Design review of the part built by this model. Coordinates are the model's own, in mm. A direction names the side the tool comes from. Coordinates: 2 decimals unless noted, no trailing zeros. Loops run counter-clockwise (first coordinate to the right, second up) from the corner with the lowest first, then second, coordinate; pieces in that order, holes last. Notation, with made-up numbers: (80, -18.75) -> (114, -18.75) arc R23 cw to (114, -2.75) -> close; hole circle Ø7 at (48, 8). An arc over 180 degrees is marked (long way). One line per item, written item: value. Start each with the question number.
1. Add section A-A on z = 11. Give the number of separate pieces and of enclosed holes in the cut face, plus the area to 3 significant figures.
2. Draft analysis for pull direction Y (two halves, no side actions). For faces 3 (the cylindrical face through (266.06, 1.81, 17.53)), 4 (the cylindrical face through (10.79, 10.89, 19.91)), 5 (the flat face through (136, 139.7, 18)), state which applies: pulls with the +Y half, pulls with the -Y half, needs draft (parallel to the pull), parting line crosses it, or undercut.
3. Add section B-B on y = 16. Write out the cut boundary in (x, z).
4. Insertion check: pin 1 (1.5 mm diameter, centred on x = 147.5, y = 18.5, fed in from +Z); pin 2 (1.5 mm diameter, centred on x = 6, z = 33.5, fed in from -Y); pin 3 (1.3 mm diameter, centred on y = 135, z = 25.5, fed in from -X); pin 4 (1.6 mm diameter, centred on x = 260.5, y = 6, fed in from +Z). Each pin has a flat end and moves straight along its axis. Give the tip position at first contact, or say it passes through.
5. For probe 1 along Y at (x, z) = (261.62, 12.5); probe 2 along Y at (x, z) = (198, 31); probe 3 along X at (y, z) = (133.35, 15.75), list the stretches that pass through material, from the lowest coordinate up.
6. Machinability: for faces 1 (the flat face through (136, 135.89, 19)), 2 (the cylindrical face through (1.91, 137.89, 17.53)), which of the approach directions +Z, -Z, +X, -X, +Y, -Y give a long, thin tool a straight path to every point of the face, cutting with its end or side? Answer none if there is none.
7. Add section C-C on x = 210. Write out the cut boundary in (y, z).
```python
from build123d import *

# Parameters (mm, degrees)
BOSS_EXTRUDE1_DEPTH = 35.56
SHELL1_T            = -3.81
BOSS_EXTRUDE2_REACH = 306.284
SKETCH2_R           = 1.5875
CUT_EXTRUDE1_DEPTH  = 5.08


with BuildPart() as part:
    # Sketch1 → Boss-Extrude1 (new body)
    with BuildSketch(Plane.XY):
        with BuildLine():
            Line((6.35, 0), (261.62, 0))
            ThreePointArc((261.62, 0), (266.110128061, 1.859871939), (267.97, 6.35))
            Line((267.97, 6.35), (267.97, 133.35))
            ThreePointArc((267.97, 133.35), (266.110128061, 137.840128061), (261.62, 139.7))
            Line((261.62, 139.7), (6.35, 139.7))
            ThreePointArc((6.35, 139.7), (1.859871939, 137.840128061), (0, 133.35))
            Line((0, 133.35), (0, 6.35))
            ThreePointArc((0, 6.35), (1.859871939, 1.859871939), (6.35, 0))
        make_face()
    extrude(amount=BOSS_EXTRUDE1_DEPTH)

    # Shell1
    shell1_openings = [part.faces().sort_by_distance(p)[0] for p in [
        (133.985, 69.85, 35.56),
    ]]
    offset(amount=SHELL1_T, openings=shell1_openings, kind=Kind.INTERSECTION)

    # Sketch2 → Boss-Extrude2 (add, up to next)
    with BuildSketch(Plane.XY.offset(35.56), mode=Mode.PRIVATE) as boss_extrude2_sk1:
        with BuildLine():
            Line((255.27, 139.7), (261.62, 139.7))
            ThreePointArc((261.62, 139.7), (266.110128061, 137.840128061), (267.97, 133.35))
            Line((267.97, 133.35), (267.97, 127))
            Line((267.97, 127), (261.62, 127))
            ThreePointArc((261.62, 127), (257.129871939, 128.859871939), (255.27, 133.35))
            Line((255.27, 133.35), (255.27, 139.7))
        make_face()
        with Locations(Location((261.62, 133.35, 0), (0, 0, 180))):
            Circle(SKETCH2_R, mode=Mode.SUBTRACT)
    boss_extrude2_tool1 = extrude(boss_extrude2_sk1.sketch, amount=-BOSS_EXTRUDE2_REACH, mode=Mode.PRIVATE) - part.part
    # Sketch2 → Boss-Extrude2 (add, up to next)
    with BuildSketch(Plane.XY.offset(35.56), mode=Mode.PRIVATE) as boss_extrude2_sk2:
        with BuildLine():
            Line((12.7, 133.35), (12.7, 139.7))
            Line((12.7, 139.7), (6.35, 139.7))
            ThreePointArc((6.35, 139.7), (1.859871939, 137.840128061), (0, 133.35))
            Line((0, 133.35), (0, 127))
            Line((0, 127), (6.35, 127))
            ThreePointArc((6.35, 127), (10.840128061, 128.859871939), (12.7, 133.35))
        make_face()
        with Locations((6.35, 133.35)):
            Circle(SKETCH2_R, mode=Mode.SUBTRACT)
    boss_extrude2_tool2 = extrude(boss_extrude2_sk2.sketch, amount=-BOSS_EXTRUDE2_REACH, mode=Mode.PRIVATE) - part.part
    # Sketch2 → Boss-Extrude2 (add, up to next)
    with BuildSketch(Plane.XY.offset(35.56), mode=Mode.PRIVATE) as boss_extrude2_sk3:
        with BuildLine():
            Line((12.7, 0), (6.35, 0))
            ThreePointArc((6.35, 0), (1.859871939, 1.859871939), (0, 6.35))
            Line((0, 6.35), (0, 12.7))
            Line((0, 12.7), (6.35, 12.7))
            ThreePointArc((6.35, 12.7), (10.840128061, 10.840128061), (12.7, 6.35))
            Line((12.7, 6.35), (12.7, 0))
        make_face()
        with Locations(Location((6.35, 6.35, 0), (0, 0, 180))):
            Circle(SKETCH2_R, mode=Mode.SUBTRACT)
    boss_extrude2_tool3 = extrude(boss_extrude2_sk3.sketch, amount=-BOSS_EXTRUDE2_REACH, mode=Mode.PRIVATE) - part.part
    # Sketch2 → Boss-Extrude2 (add, up to next)
    with BuildSketch(Plane.XY.offset(35.56), mode=Mode.PRIVATE) as boss_extrude2_sk4:
        with BuildLine():
            Line((255.27, 6.35), (255.27, 0))
            Line((255.27, 0), (261.62, 0))
            ThreePointArc((261.62, 0), (266.110128061, 1.859871939), (267.97, 6.35))
            Line((267.97, 6.35), (267.97, 12.7))
            Line((267.97, 12.7), (261.62, 12.7))
            ThreePointArc((261.62, 12.7), (257.129871939, 10.840128061), (255.27, 6.35))
        make_face()
        with Locations((261.62, 6.35)):
            Circle(SKETCH2_R, mode=Mode.SUBTRACT)
    boss_extrude2_tool4 = extrude(boss_extrude2_sk4.sketch, amount=-BOSS_EXTRUDE2_REACH, mode=Mode.PRIVATE) - part.part
    add(boss_extrude2_tool1.solids().sort_by_distance((258.445, 139.520395, 35.56))[0])
    add(boss_extrude2_tool2.solids().sort_by_distance((12.520395, 136.525, 35.56))[0])
    add(boss_extrude2_tool3.solids().sort_by_distance((12.520395, 3.175, 35.56))[0])
    add(boss_extrude2_tool4.solids().sort_by_distance((257.256872, 10.713128, 35.56))[0])

    # Sketch3 → Cut-Extrude1 (cut)
    with BuildSketch(Plane.XY.offset(35.56)):
        Polygon((9.398, 133.35), (7.874, 135.989645431), (4.826, 135.989645431), (3.302, 133.35), (4.826, 130.710354569), (7.874, 130.710354569), align=None)
        Polygon((258.572, 133.35), (260.096, 130.710354569), (263.144, 130.710354569), (264.668, 133.35), (263.144, 135.989645431), (260.096, 135.989645431), align=None)
        Polygon((264.668, 6.35), (263.144, 8.989645431), (260.096, 8.989645431), (258.572, 6.35), (260.096, 3.710354569), (263.144, 3.710354569), align=None)
        Polygon((9.398, 6.35), (7.874, 8.989645431), (4.826, 8.989645431), (3.302, 6.35), (4.826, 3.710354569), (7.874, 3.710354569), align=None)
    extrude(amount=-CUT_EXTRUDE1_DEPTH, mode=Mode.SUBTRACT)


solid = part.part
```
Worked answers:
1. separate pieces: 1
1. enclosed holes: 5
1. area: 3,260 mm²
2. face 3: pulls with the -Y half
2. face 4: undercut
2. face 5: pulls with the +Y half
3. outline: (0, 0) -> (267.97, 0) -> (267.97, 35.56) -> (264.16, 35.56) -> (264.16, 3.81) -> (3.81, 3.81) -> (3.81, 35.56) -> (0, 35.56) -> close
4. pin 1: stops at z = 3.81
4. pin 2: stops at y = 0
4. pin 3: stops at x = 0.08
4. pin 4: stops at z = 30.48
5. probe 1: y = 0 to 4.76, 7.94 to 12.7, 127 to 131.76, 134.94 to 139.7
5. probe 2: y = 0 to 3.81, 135.89 to 139.7
5. probe 3: x = 0 to 4.76, 7.94 to 12.7, 255.27 to 260.03, 263.21 to 267.97
6. face 1: +Z
6. face 2: +Z, -Z, -X, +Y
7. outline: (0, 0) -> (139.7, 0) -> (139.7, 35.56) -> (135.89, 35.56) -> (135.89, 3.81) -> (3.81, 3.81) -> (3.81, 35.56) -> (0, 35.56) -> close
